Could you check a few things on this drawing? It's one solid part, dimensions in mm from its lowest x, y, z. A direction names the side the tool comes from. Round coordinates to 2 decimals unless told otherwise and drop trailing zeros. Write each loop counter-clockwise with the first axis right and the second up, starting at its lowest first coordinate (ties: lowest second). Pieces come first, ordered by that corner, then holes. Notation, with made-up numbers: (-12, -20.5) -> (33, -20.5) arc R24 ccw to (33, -1.5) -> close; hole circle Ø1 at (32, 53). An arc over 180 degrees is marked (long way). Return JSON: item names as keys, results as strings.
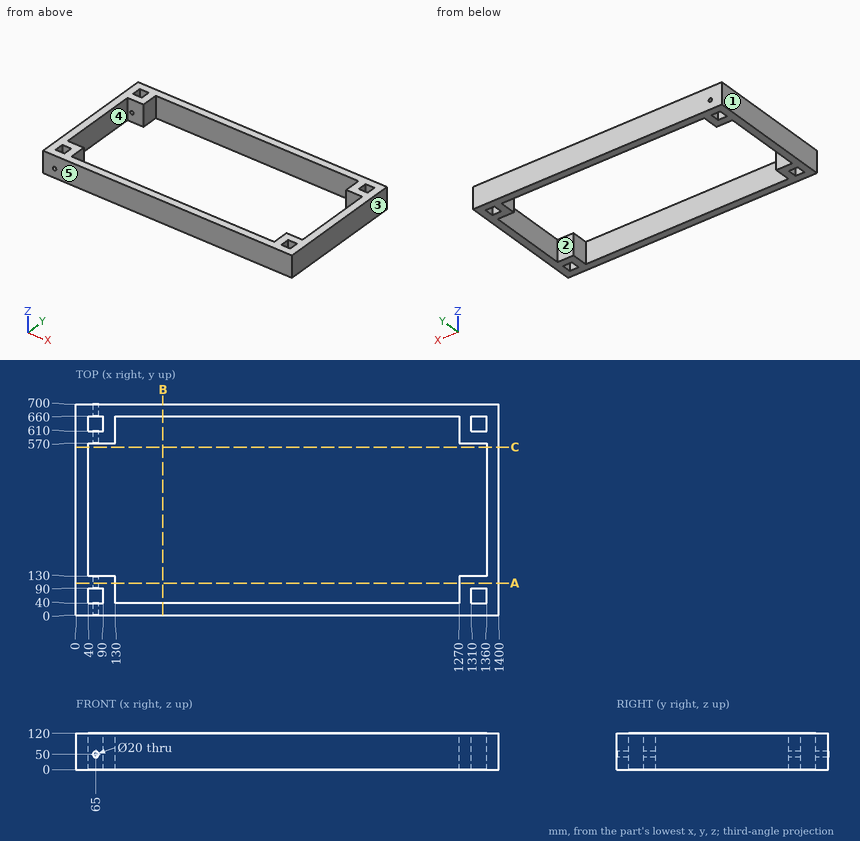
1) I want a section at C-C, the plane y = 557. Please give me the cut outline in (x, z).
Return value:
{"outline": "(0, 0) -> (40, 0) -> (40, 120) -> (0, 120) -> close; (1360, 0) -> (1400, 0) -> (1400, 120) -> (1360, 120) -> close"}
2) If I drill on probe 1 along X at (y, z) = (83, 68.5); probe 2 along X at (y, z) = (348.5, 10.5); probe 3 along Y at (x, z) = (827, 106), over which ranges is the centre line in solid material (lowest first)? Write a range as [from, to].
Return value:
{"probe 1": "[0, 40], [90, 130], [1270, 1310], [1360, 1400]", "probe 2": "[0, 40], [1360, 1400]", "probe 3": "[0, 40], [660, 700]"}
3) For the marked faces 4 and 5, which set-ups out of +Z, -Z, +X, -X, +Y, -Y let a thin tool reach every point of the face, with its end or its side?
Return value:
{"face 4": "+Z, -Z", "face 5": "+Z, -Z, +X, -X, -Y"}
4) Thinking about a two-plate mould opening in X: for the marked faces 1, 2 and 3, which applies, pulls with the +X half, pulls with the -X half, needs draft (parallel to the pull), parting line crosses it, or undercut?
Return value:
{"face 1": "pulls with the -X half", "face 2": "undercut", "face 3": "pulls with the +X half"}
5) I want a section at A-A, the plane y = 107. Please give me the cut outline in (x, z).
Return value:
{"outline": "(0, 0) -> (130, 0) -> (130, 120) -> (0, 120) -> close; (1270, 0) -> (1400, 0) -> (1400, 120) -> (1270, 120) -> close; hole circle Ø20 at (65, 50)"}
6) I want a section at B-B, the plane x = 287.5. Please give me the cut outline in (y, z).
Return value:
{"outline": "(0, 0) -> (40, 0) -> (40, 120) -> (0, 120) -> close; (660, 0) -> (700, 0) -> (700, 120) -> (660, 120) -> close"}
